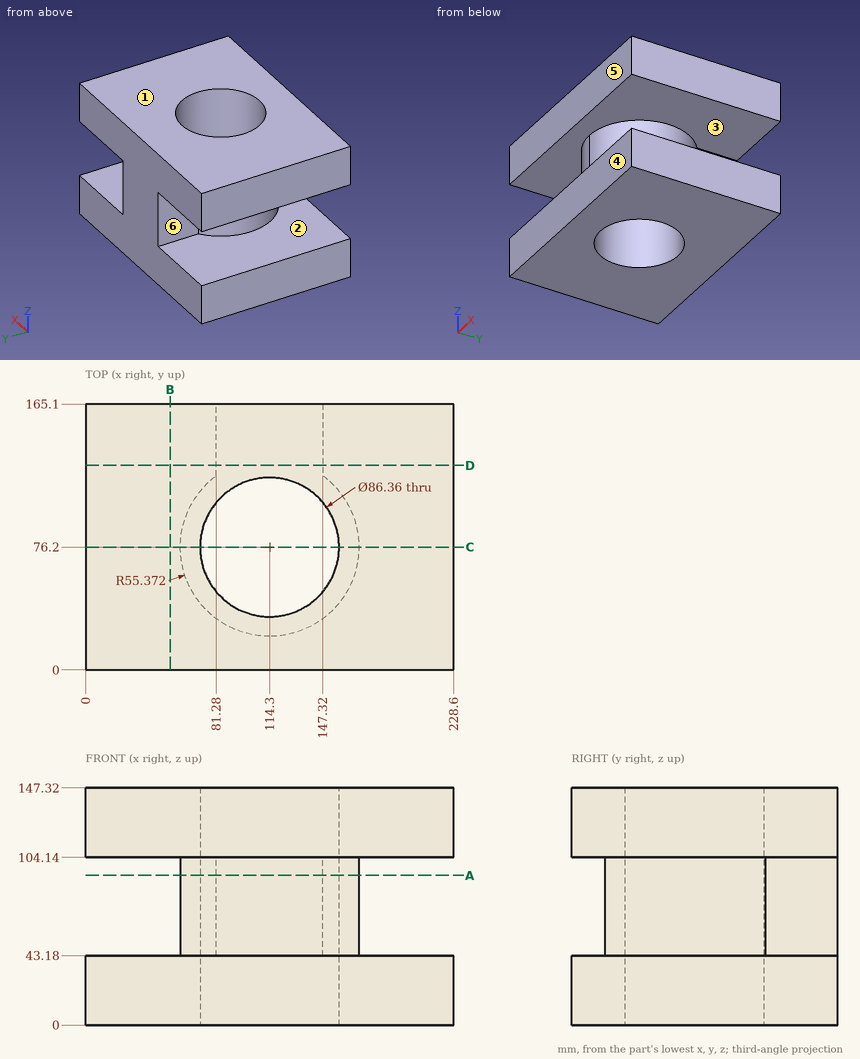
Geometry check sheet. Reference: drawing and pictorial views, mm from the part's lowest x, y, z. A direction names the side the tool comes from. Coordinates: 2 decimals unless noted, no trailing zeros. Write each loop counter-clockwise with the first axis right and the second up, starting at its lowest first coordinate (ties: lowest second). Pieces come first, ordered by that corner, then holes. Notation, with made-up numbers: (33, 33.25) -> (76, 33.25) arc R33 cw to (76, 63.25) -> close; hole circle Ø3 at (-21, -1). An arc over 180 degrees is marked (long way). Use a Markdown table: item, result.
1. Scan lines: line 1 along Z through (x, y) = (28.5, 96); line 2 along X through (y, z) = (76, 85); line 3 along Y through (x, z) = (114, 69). Record each from-to range of solid material in increasing order.
Reported:
| item | result |
|---|---|
| line 1 | z = 0 to 43.18, 104.14 to 147.32 |
| line 2 | x = 58.93 to 71.12, 157.48 to 169.67 |
| line 3 | y = 20.83 to 33.02, 119.38 to 165.1 |
2. Sectioned sample at C-C (y = 76.2). Enter the section's corners in (x, z), plus the area to 3 significant figures.
Reported:
| item | result |
|---|---|
| outline | (0, 0) -> (71.12, 0) -> (71.12, 147.32) -> (0, 147.32) -> (0, 104.14) -> (58.93, 104.14) -> (58.93, 43.18) -> (0, 43.18) -> close; (157.48, 0) -> (228.6, 0) -> (228.6, 43.18) -> (169.67, 43.18) -> (169.67, 104.14) -> (228.6, 104.14) -> (228.6, 147.32) -> (157.48, 147.32) -> close |
| area | 13,800 mm2 |
3. Release check for a two-part mould opening along Z. For the marked faces 1, 2, 3 and 4 record: pulls with the +Z half, pulls with the -Z half, needs draft (parallel to the pull), parting line crosses it, or undercut.
Reported:
| item | result |
|---|---|
| face 1 | pulls with the +Z half |
| face 2 | undercut |
| face 3 | undercut |
| face 4 | needs draft |
4. Sectioned sample at D-D (y = 127). Enter the section's corners in (x, z), plus the area to 3 significant figures.
Reported:
| item | result |
|---|---|
| outline | (0, 0) -> (228.6, 0) -> (228.6, 43.18) -> (147.32, 43.18) -> (147.32, 104.14) -> (228.6, 104.14) -> (228.6, 147.32) -> (0, 147.32) -> (0, 104.14) -> (81.28, 104.14) -> (81.28, 43.18) -> (0, 43.18) -> close |
| area | 23,800 mm2 |
5. Tool access check on the marked faces 5 and 6. Record the directions out of +Z, -Z, +X, -X, +Y, -Y that give a thin tool (end or side, any length) a straight path to the whole face; none if there is none.
Reported:
| item | result |
|---|---|
| face 5 | +Z, -Z, +X, -X, -Y |
| face 6 | -X, +Y |
6. Go/stop test with flat-tipped pins: pin 1 Ø6 at (x, z) = (75, 106) entering from -Y; pin 2 Ø10 at (y, z) = (80, 74.5) entering from +X; pin 3 Ø5 at (y, z) = (24.5, 56.5) entering from +X; pin 4 Ø13.5 at (y, z) = (143, 73.5) entering from +X. Record where each tip stops, or that it passes through.
Reported:
| item | result |
|---|---|
| pin 1 | stops at y = 0 |
| pin 2 | stops at x = 169.67 |
| pin 3 | stops at x = 139.71 |
| pin 4 | stops at x = 147.32 |
7. Sectioned sample at A-A (z = 93). Enter the section's corners in (x, y), plus the area to 3 significant figures.
Reported:
| item | result |
|---|---|
| outline | (81.28, 120.65) arc R55.37 ccw (long way) to (147.32, 120.65) -> (147.32, 165.1) -> (81.28, 165.1) -> close; hole circle Ø86.36 at (114.3, 76.2) |
| area | 6,220 mm2 |
8. Sectioned sample at B-B (x = 52.5). Enter the section's corners in (y, z), plus the area to 3 significant figures.
Reported:
| item | result |
|---|---|
| outline | (0, 0) -> (165.1, 0) -> (165.1, 43.18) -> (0, 43.18) -> close; (0, 104.14) -> (165.1, 104.14) -> (165.1, 147.32) -> (0, 147.32) -> close |
| area | 14,300 mm2 |
